```python
from build123d import *

# Parameters (mm, degrees)
BOSS_EXTRUDE1_DEPTH      = 1
SKETCH2_R                = 1.325
CUT_EXTRUDE1_DEPTH       = 36.80851854
SKETCH3_R                = 0.5
CUT_EXTRUDE2_DEPTH       = 36.80851854
LPATTERN1_COUNT          = 20
LPATTERN1_PITCH          = 2.54
BOSS_EXTRUDE6_DEPTH      = 1.25
BOSS_EXTRUDE6_DEPTH_BACK = 4.5
CUT_EXTRUDE9_DEPTH       = 5.25
SKETCH_1_W               = 4.7
SKETCH_1_H               = 2.3
EXTRUDE_1_DEPTH          = 2
SKETCH_2_W               = 1.86
SKETCH_2_H               = 1
EXTRUDE_2_DEPTH          = 1
SKETCH_6_W               = 6.64
SKETCH_6_H               = 3
EXTRUDE_6_DEPTH          = 1.36
SKETCH_7_W               = 2.5
SKETCH_7_H               = 1
CUT_EXTRUDE_1_DEPTH      = 0.1
SKETCH_8_W               = 1.3
SKETCH_8_H               = 1
EXTRUDE_7_DEPTH          = 1.6
SKETCH_9_R               = 2.75
SKETCH_9_R_2             = 1.325
EXTRUDE_8_DEPTH          = 1.5
SKETCH_10_R              = 1.05
EXTRUDE_9_DEPTH          = 2.5
SKETCH_11_R              = 0.5
EXTRUDE_10_DEPTH         = 3


with BuildPart() as part:
    # Sketch1 → Boss-Extrude1 (new body)
    with BuildSketch(Plane(origin=(0, 0, 0), x_dir=(1, 0, 0), z_dir=(0, 1, 0))):
        with BuildLine():
            Line((-28.75, 15), (28.75, 15))
            ThreePointArc((28.75, 15), (31.401650429, 13.901650429), (32.5, 11.25))
            Line((32.5, 11.25), (32.5, -11.25))
            ThreePointArc((32.5, -11.25), (31.401650429, -13.901650429), (28.75, -15))
            Line((28.75, -15), (-28.75, -15))
            ThreePointArc((-28.75, -15), (-31.401650429, -13.901650429), (-32.5, -11.25))
            Line((-32.5, -11.25), (-32.5, 11.25))
            ThreePointArc((-32.5, 11.25), (-31.401650429, 13.901650429), (-28.75, 15))
        make_face()
    extrude(amount=BOSS_EXTRUDE1_DEPTH)

    # Sketch2 → Cut-Extrude1 (cut, through all)
    with BuildSketch(Plane(origin=(0, 1, 0), x_dir=(1, 0, 0), z_dir=(0, 1, 0))):
        with Locations(Location((-29.025, 11.525, 0), (0, 0, 270))):
            Circle(SKETCH2_R)
        with Locations(Location((29.025, 11.525, 0), (0, 0, 90))):
            Circle(SKETCH2_R)
        with Locations(Location((29.025, -11.525, 0), (0, 0, 270))):
            Circle(SKETCH2_R)
        with Locations(Location((-29.025, -11.525, 0), (0, 0, 90))):
            Circle(SKETCH2_R)
    extrude(amount=-CUT_EXTRUDE1_DEPTH, mode=Mode.SUBTRACT)

    # Sketch3 → Cut-Extrude2 (cut, through all)
    with BuildSketch(Plane(origin=(0, 1, 0), x_dir=(1, 0, 0), z_dir=(0, 1, 0))):
        with Locations(Location((-24.128, 13, 0), (0, 0, 270))):
            Circle(SKETCH3_R)
        with Locations(Location((-24.128, 10.5, 0), (0, 0, 270))):
            Circle(SKETCH3_R)
    cut_extrude2 = extrude(amount=-CUT_EXTRUDE2_DEPTH, mode=Mode.SUBTRACT)

    # LPattern1: Cut-Extrude2 ×20
    with Locations(*[(i * LPATTERN1_PITCH, 0, 0) for i in range(1, LPATTERN1_COUNT)]):
        add(cut_extrude2, mode=Mode.SUBTRACT)

    # Sketch15 → Boss-Extrude6 (add, two sides: drawn at the far end of the back side and taken through both)
    with BuildSketch(Plane.XY.offset(15).offset(-BOSS_EXTRUDE6_DEPTH_BACK)):
        with BuildLine():
            Line((-24.6, 3.6), (-17.85, 3.6))
            ThreePointArc((-17.85, 3.6), (-17.567157288, 3.482842712), (-17.45, 3.2))
            Line((-17.45, 3.2), (-17.45, 2.652310288))
            ThreePointArc((-17.45, 2.652310288), (-17.522264229, 2.279072643), (-17.728612679, 1.959778459))
            Line((-17.728612679, 1.959778459), (-18.354830555, 1.307468172))
            ThreePointArc((-18.354830555, 1.307468172), (-18.684128491, 1.080072876), (-19.076217876, 1))
            Line((-19.076217876, 1), (-23.373782124, 1))
            ThreePointArc((-23.373782124, 1), (-23.765871509, 1.080072876), (-24.095169445, 1.307468172))
            Line((-24.095169445, 1.307468172), (-24.721387321, 1.959778459))
            ThreePointArc((-24.721387321, 1.959778459), (-24.927735771, 2.279072643), (-25, 2.652310288))
            Line((-25, 2.652310288), (-25, 3.2))
            ThreePointArc((-25, 3.2), (-24.882842712, 3.482842712), (-24.6, 3.6))
        make_face()
    extrude(amount=BOSS_EXTRUDE6_DEPTH + BOSS_EXTRUDE6_DEPTH_BACK)

    # Sketch16 → Cut-Extrude9 (cut)
    with BuildSketch(Plane.XY.offset(16.25)):
        with BuildLine():
            Line((-18.585674498, 1.529078357), (-17.959456622, 2.181388644))
            ThreePointArc((-17.959456622, 2.181388644), (-17.819139676, 2.398508689), (-17.77, 2.652310288))
            Line((-17.77, 2.652310288), (-17.77, 3.2))
            ThreePointArc((-17.77, 3.2), (-17.793431458, 3.256568542), (-17.85, 3.28))
            Line((-17.85, 3.28), (-24.6, 3.28))
            ThreePointArc((-24.6, 3.28), (-24.656568542, 3.256568542), (-24.68, 3.2))
            Line((-24.68, 3.2), (-24.68, 2.652310288))
            ThreePointArc((-24.68, 2.652310288), (-24.630860324, 2.398508689), (-24.490543378, 2.181388644))
            Line((-24.490543378, 2.181388644), (-23.864325502, 1.529078357))
            ThreePointArc((-23.864325502, 1.529078357), (-23.640402906, 1.374449555), (-23.373782124, 1.32))
            Line((-23.373782124, 1.32), (-19.076217876, 1.32))
            ThreePointArc((-19.076217876, 1.32), (-18.809597094, 1.374449555), (-18.585674498, 1.529078357))
        make_face()
    extrude(amount=-CUT_EXTRUDE9_DEPTH, mode=Mode.SUBTRACT)

    # 草图1 → 凸台-拉伸1 (add)
    with BuildSketch(Plane(origin=(0, 1, 0), x_dir=(1, 0, 0), z_dir=(0, 1, 0))):
        with Locations((-10.52, -13.05)):
            Rectangle(SKETCH_1_W, SKETCH_1_H)
    extrude(amount=EXTRUDE_1_DEPTH)

    # 草图2 → 凸台-拉伸2 (add)
    with BuildSketch(Plane.XY.offset(14.2)):
        with Locations((-10.52, 2)):
            Rectangle(SKETCH_2_W, SKETCH_2_H)
    extrude(amount=EXTRUDE_2_DEPTH)

    # 草图6 → 凸台-拉伸6 (add)
    with BuildSketch(Plane(origin=(0, 1, 0), x_dir=(1, 0, 0), z_dir=(0, 1, 0))):
        with Locations((20.35, -12.9)):
            Rectangle(SKETCH_6_W, SKETCH_6_H)
    extrude(amount=EXTRUDE_6_DEPTH)

    # 草图7 → 切除-拉伸1 (cut)
    with BuildSketch(Plane.XY.offset(14.4)):
        with Locations((20.35, 1.86)):
            Rectangle(SKETCH_7_W, SKETCH_7_H)
    extrude(amount=-CUT_EXTRUDE_1_DEPTH, mode=Mode.SUBTRACT)

    # 草图8 → 凸台-拉伸7 (add)
    with BuildSketch(Plane.XY.offset(14.3)):
        with Locations((19.75, 1.86)):
            Rectangle(SKETCH_8_W, SKETCH_8_H)
    extrude(amount=EXTRUDE_7_DEPTH)

    # 草图9 → 凸台-拉伸8 (add)
    # profile 1 of 4: a face of its own
    with BuildSketch(Plane.XZ):
        with Locations(Location((29.025, 11.525, 0), (0, 0, 90))):
            Circle(SKETCH_9_R)
        with Locations(Location((29.025, 11.525, 0), (0, 0, 90))):
            Circle(SKETCH_9_R_2, mode=Mode.SUBTRACT)
    # profile 2 of 4: a face of its own
    with BuildSketch(Plane.XZ):
        with Locations(Location((29.025, -11.525, 0), (0, 0, 90))):
            Circle(SKETCH_9_R)
        with Locations(Location((29.025, -11.525, 0), (0, 0, 270))):
            Circle(SKETCH_9_R_2, mode=Mode.SUBTRACT)
    # profile 3 of 4: a face of its own
    with BuildSketch(Plane.XZ):
        with Locations(Location((-29.025, 11.525, 0), (0, 0, 90))):
            Circle(SKETCH_9_R)
        with Locations(Location((-29.025, 11.525, 0), (0, 0, 270))):
            Circle(SKETCH_9_R_2, mode=Mode.SUBTRACT)
    # profile 4 of 4: a face of its own
    with BuildSketch(Plane.XZ):
        with Locations(Location((-29.025, -11.525, 0), (0, 0, 90))):
            Circle(SKETCH_9_R)
        with Locations(Location((-29.025, -11.525, 0), (0, 0, 90))):
            Circle(SKETCH_9_R_2, mode=Mode.SUBTRACT)
    extrude(amount=EXTRUDE_8_DEPTH)

    # 草图10 → 凸台-拉伸9 (add)
    with BuildSketch(Plane(origin=(0, 1, 0), x_dir=(1, 0, 0), z_dir=(0, 1, 0))):
        with Locations(Location((24.132, 13, 0), (0, 0, 270))):
            Circle(SKETCH_10_R)
        with Locations(Location((21.592, 13, 0), (0, 0, 270))):
            Circle(SKETCH_10_R)
        with Locations(Location((19.052, 13, 0), (0, 0, 270))):
            Circle(SKETCH_10_R)
        with Locations(Location((21.592, 10.5, 0), (0, 0, 270))):
            Circle(SKETCH_10_R)
        with Locations(Location((19.052, 10.5, 0), (0, 0, 270))):
            Circle(SKETCH_10_R)
        with Locations(Location((-24.128, 10.5, 0), (0, 0, 270))):
            Circle(SKETCH_10_R)
    extrude(amount=EXTRUDE_9_DEPTH)

    # 草图11 → 凸台-拉伸10 (add)
    with BuildSketch(Plane.XZ.offset(-1)):
        with Locations(Location((24.132, -13, 0), (0, 0, 90))):
            Circle(SKETCH_11_R)
        with Locations(Location((21.592, -13, 0), (0, 0, 90))):
            Circle(SKETCH_11_R)
        with Locations(Location((21.592, -10.5, 0), (0, 0, 90))):
            Circle(SKETCH_11_R)
        with Locations(Location((19.052, -10.5, 0), (0, 0, 90))):
            Circle(SKETCH_11_R)
        with Locations(Location((19.052, -13, 0), (0, 0, 90))):
            Circle(SKETCH_11_R)
        with Locations(Location((-24.128, -10.5, 0), (0, 0, 90))):
            Circle(SKETCH_11_R)
    extrude(amount=EXTRUDE_10_DEPTH)


solid = part.part
```
Part model, mm, in its own coordinate system. A direction names the side the tool comes from. Round coordinates to 2 decimals unless told otherwise and drop trailing zeros. Write each loop counter-clockwise with the first axis right and the second up, starting at its lowest first coordinate (ties: lowest second). Pieces come first, ordered by that corner, then holes. Notation, with made-up numbers: M -29,29 L -20,29 A9 cw -20,40 Z; hole C -15.5,51 d3. An arc over 180 degrees is marked long. Answer as CSV lines item,"result". Start each with the question number.
1) Which spindle directions (+Z, -Z, +X, -X, +Y, -Y) get a long thin tool onto all of the face, cutting with end or side? Do faces 1 (the face through (-21, 1, 16)), 2 (the face through (-11, 2, 11.9)), 3 (the face through (-12.87, 2, 13)), 4 (the face through (-24, 3.5, -11)), 5 (the face through (-31.75, -0.74, 11.17)). Say none if no direction does.
2) Band-saw the part on A-A (z = 6.5). List the corners of the cut face in (x, y), then the cut area to 3 significant figures.
3) Drop flat-ended pins along their axis: pin 1 (0.8 mm diameter, centred on y = 2, z = 14.5, fed in from +X); pin 2 (0.6 mm diameter, centred on x = -10, y = 1.5, fed in from +Z); pin 3 (1.4 mm diameter, centred on x = 20, z = 15, fed in from -Y). Give the stop position or say it passes through.
4) Mould opens along X. For faces 6 (the face through (-31.75, -0.74, -11.88)), 7 (the face through (-30, -1.5, -10)) say: +X half, -X half, draft (parallel to the pull), parting line (faces both ways), or undercut.
5) Drill centre lines: L1, parallel to Z at x = -9, y = 0.3; L2, parallel to X at y = -1.4, z = 10.5; L3, parallel to Y at x = 29.5, z = 1.5. Where is each one in solid material? Low to high.
Worked out:
1,face 1,"+Z, +X, -X, -Y"
1,face 2,"-Z, +Y"
1,face 3,"+Z, -Z, +Y"
1,face 4,"-Z, +X, -X, +Y"
1,face 5,"-Y"
2,outline,"M -32.5,0 L 32.5,0 L 32.5,1 L -32.5,1 Z"
2,area,"65.0 mm²"
3,pin 1,"x = 23.67"
3,pin 2,"z = 15.2"
3,pin 3,"y = 0"
4,face 6,"undercut"
4,face 7,"draft"
5,L1,"-15 to -13.49, -12.51 to -10.99, -10.01 to 15"
5,L2,"-31.58 to -29.86, -28.19 to -26.47, 26.47 to 28.19, 29.86 to 31.58"
5,L3,"0 to 1"
